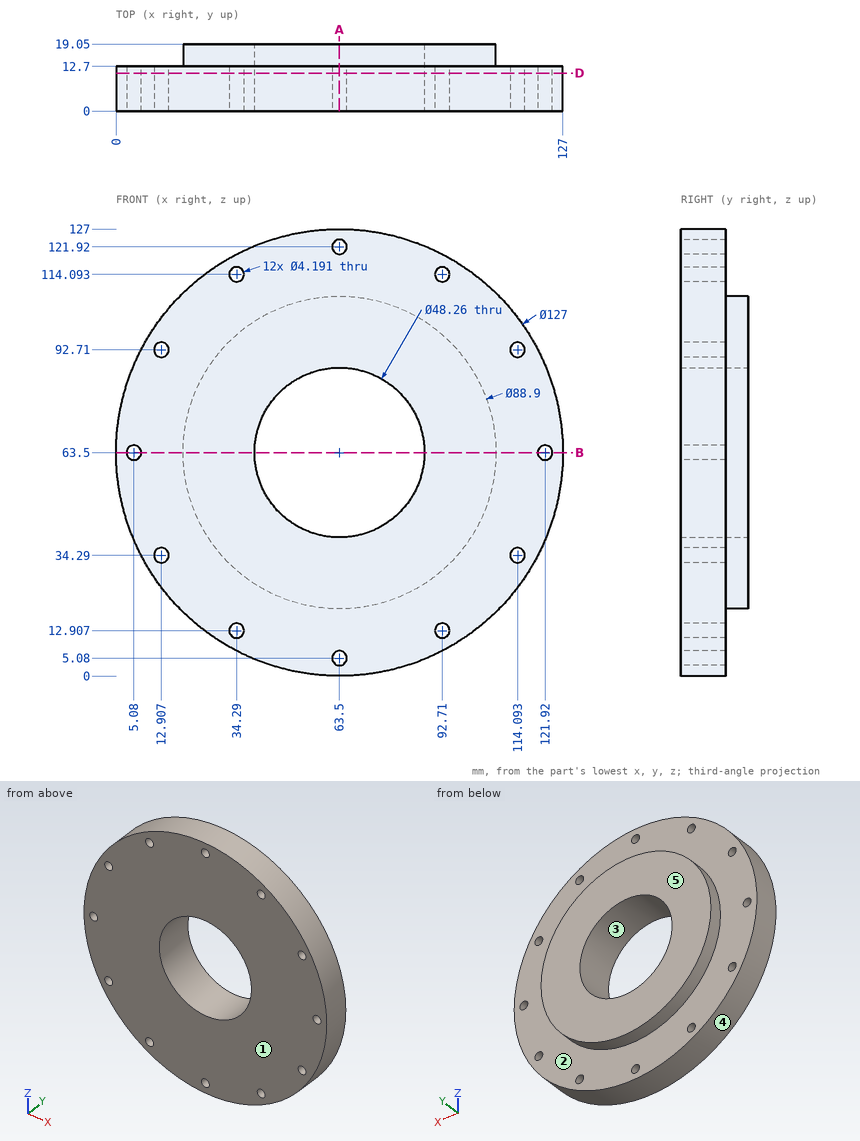
Study the drawing (mm; zero at the part's minimum x, y, z) and answer. A direction names the side the tool comes from. Give positions to 0.01 mm unless a question says otherwise; leave off trailing zeros. Write each loop counter-clockwise with the first axis right and the second up, starting at its lowest first coordinate (ties: lowest second). Pieces come first, ordered by that corner, then holes. Notation, with made-up numbers: (76, -3) - (106, -3) arc R16 ccw to (106, 24) - close; hole circle Ø6 at (3.25, -11). An arc over 180 degrees is marked (long way). Write item = value, one per line. Start each with the question number.
Item 1: Each of these flat-tipped pins is pushed along its axis until it touches: P1, Ø3, axis at x = 94.5, z = 25.5, coming from the +Y side; P2, Ø3, axis at x = 41.5, y = 11.5, coming from the -Z side; P3, Ø10, axis at x = 87, y = 9.5, coming from the -Z side (1 decimal). Where does it stop, or does it pass through?
Item 2: Find section D-D (y = 10.75). State how many separate pieces and enclosed holes the cut face has, then the cut area to 3 significant figures.
Item 3: Find the intervals of material crossed by probe 1 along Z at (x, y) = (92.71, 7); probe 2 along Y at (x, z) = (30, 108); probe 3 along Z at (x, y) = (70.5, 1.75), in increasing order. Write a range as [from, to].
Item 4: A tool of negligible diameter and unlimited length cuts with its end or side. For the marked faces 1 and 2, from which of +Z, -Z, +X, -X, +Y, -Y can it reach the whole face along a straight path? Write none if from no direction.
Item 5: Find section A-A (x = 63.5). Give the vertices of the cut face in (y, z), then the cut area to 3 significant figures.
Item 6: Find section B-B (z = 63.5). Give the vertices of the cut face in (x, y).
Item 7: The mould has two halves that part along X. Classify the marked faces 3, 4 and 5: +X half, -X half, draft (parallel to the pull), parting line (faces both ways), or undercut.
Response:
q1.P1 = 12.7
q1.P2 = 3.4
q1.P3 = 2.8
q2.separate_pieces = 1
q2.enclosed_holes = 13
q2.area = 10,700 mm²
q3.probe_1 = [7.12, 10.81], [15, 112], [116.19, 119.88]
q3.probe_2 = [0, 12.7]
q3.probe_3 = [0.39, 40.41], [86.59, 126.61]
q4.face_1 = +Z, -Z, +X, -X, -Y
q4.face_2 = +Y
q5.outline = (0, 0) - (12.7, 0) - (12.7, 2.98) - (0, 2.98) - close; (0, 7.18) - (12.7, 7.18) - (12.7, 19.05) - (19.05, 19.05) - (19.05, 39.37) - (0, 39.37) - close; (0, 87.63) - (19.05, 87.63) - (19.05, 107.95) - (12.7, 107.95) - (12.7, 119.82) - (0, 119.82) - close; (0, 124.02) - (12.7, 124.02) - (12.7, 127) - (0, 127) - close
q5.area = 1,150 mm²
q6.outline = (0, 0) - (2.98, 0) - (2.98, 12.7) - (0, 12.7) - close; (7.18, 0) - (39.37, 0) - (39.37, 19.05) - (19.05, 19.05) - (19.05, 12.7) - (7.18, 12.7) - close; (87.63, 0) - (119.82, 0) - (119.82, 12.7) - (107.95, 12.7) - (107.95, 19.05) - (87.63, 19.05) - close; (124.02, 0) - (127, 0) - (127, 12.7) - (124.02, 12.7) - close
q7.face_3 = undercut
q7.face_4 = parting line
q7.face_5 = draft
